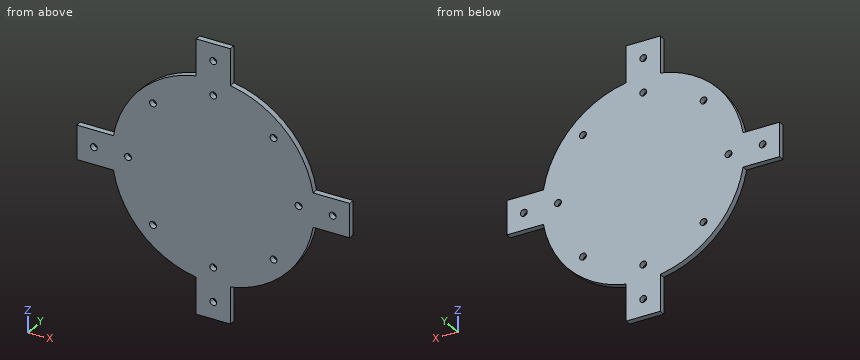
```python
from build123d import *

# Parameters (mm, degrees)
SALIENTE_EXTRUIR1_DEPTH = 3.5
CROQUIS2_R              = 2
CORTAR_EXTRUIR1_DEPTH   = 3.5
MATRIZC1_COUNT          = 8
CORTAR_EXTRUIR2_REACH   = 5.5
CROQUIS4_R              = 2


with BuildPart() as part:
    # Croquis1 → Saliente-Extruir1 (new body)
    with BuildSketch(Plane(origin=(0, 0, 0), x_dir=(1, 0, 0), z_dir=(0, 1, 0))):
        with BuildLine():
            Line((-10, -58.530413525), (-10, -80))
            Line((-10, -80), (10, -80))
            Line((10, -80), (10, -58.530413525))
            ThreePointArc((10, -58.530413525), (41.986958138, -41.986958138), (58.530413525, -10))
            Line((58.530413525, -10), (80, -10))
            Line((80, -10), (80, 10))
            Line((80, 10), (58.530413525, 10))
            ThreePointArc((58.530413525, 10), (41.986958138, 41.986958138), (10, 58.530413525))
            Line((10, 58.530413525), (10, 80))
            Line((10, 80), (-10, 80))
            Line((-10, 80), (-10, 58.530413525))
            ThreePointArc((-10, 58.530413525), (-41.986958138, 41.986958138), (-58.530413525, 10))
            Line((-58.530413525, 10), (-80, 10))
            Line((-80, 10), (-80, -10))
            Line((-80, -10), (-58.530413525, -10))
            ThreePointArc((-58.530413525, -10), (-41.986958138, -41.986958138), (-10, -58.530413525))
        make_face()
    extrude(amount=SALIENTE_EXTRUIR1_DEPTH)

    # Croquis2 → Cortar-Extruir1 (cut)
    with BuildSketch(Plane(origin=(0, 3.5, 0), x_dir=(1, 0, 0), z_dir=(0, 1, 0))):
        with Locations((0, 50)):
            Circle(CROQUIS2_R)
    cortar_extruir1 = extrude(amount=-CORTAR_EXTRUIR1_DEPTH, mode=Mode.SUBTRACT)

    # MatrizC1: Cortar-Extruir1 ×8 about axis
    matrizc1_axis = Axis((0, 0, 0), (0, 1, 0))
    for i in range(1, MATRIZC1_COUNT):
        add(cortar_extruir1.rotate(matrizc1_axis, i * 360 / MATRIZC1_COUNT), mode=Mode.SUBTRACT)

    # Croquis4 → Cortar-Extruir2 (cut, up to next)
    with BuildSketch(Plane(origin=(0, 3.5, 0), x_dir=(1, 0, 0), z_dir=(0, 1, 0)), mode=Mode.PRIVATE) as cortar_extruir2_sk1:
        with Locations((0, 70)):
            Circle(CROQUIS4_R)
    cortar_extruir2_tool1 = extrude(cortar_extruir2_sk1.sketch, amount=-CORTAR_EXTRUIR2_REACH, mode=Mode.PRIVATE) & part.part
    add(cortar_extruir2_tool1.solids().sort_by_distance((0, 3.5, -70))[0], mode=Mode.SUBTRACT)
    # Croquis4 → Cortar-Extruir2 (cut, up to next)
    with BuildSketch(Plane(origin=(0, 3.5, 0), x_dir=(1, 0, 0), z_dir=(0, 1, 0)), mode=Mode.PRIVATE) as cortar_extruir2_sk2:
        with Locations((70, 0)):
            Circle(CROQUIS4_R)
    cortar_extruir2_tool2 = extrude(cortar_extruir2_sk2.sketch, amount=-CORTAR_EXTRUIR2_REACH, mode=Mode.PRIVATE) & part.part
    add(cortar_extruir2_tool2.solids().sort_by_distance((70, 3.5, 0))[0], mode=Mode.SUBTRACT)
    # Croquis4 → Cortar-Extruir2 (cut, up to next)
    with BuildSketch(Plane(origin=(0, 3.5, 0), x_dir=(1, 0, 0), z_dir=(0, 1, 0)), mode=Mode.PRIVATE) as cortar_extruir2_sk3:
        with Locations((0, -70)):
            Circle(CROQUIS4_R)
    cortar_extruir2_tool3 = extrude(cortar_extruir2_sk3.sketch, amount=-CORTAR_EXTRUIR2_REACH, mode=Mode.PRIVATE) & part.part
    add(cortar_extruir2_tool3.solids().sort_by_distance((0, 3.5, 70))[0], mode=Mode.SUBTRACT)
    # Croquis4 → Cortar-Extruir2 (cut, up to next)
    with BuildSketch(Plane(origin=(0, 3.5, 0), x_dir=(1, 0, 0), z_dir=(0, 1, 0)), mode=Mode.PRIVATE) as cortar_extruir2_sk4:
        with Locations((-70, 0)):
            Circle(CROQUIS4_R)
    cortar_extruir2_tool4 = extrude(cortar_extruir2_sk4.sketch, amount=-CORTAR_EXTRUIR2_REACH, mode=Mode.PRIVATE) & part.part
    add(cortar_extruir2_tool4.solids().sort_by_distance((-70, 3.5, 0))[0], mode=Mode.SUBTRACT)


solid = part.part
```
Model file for the job. Use its own axes, mm. Round coordinates to 2 decimals unless told otherwise and drop trailing zeros. Write each loop counter-clockwise with the first axis right and the second up, starting at its lowest first coordinate (ties: lowest second). Pieces come first, ordered by that corner, then holes. Notation, with made-up numbers: M 47.25,-13 L 75.25,-13 A14 cw 75.25,4 Z; hole C -8.75,74.5 d5. An arc over 180 degrees is marked long. Put each result on its own line as item: value.
Item 1: Flat gauge pins, fed straight in: P1, Ø3.5, axis at x = -35.36, z = 35.36, coming from the -Y side; P2, Ø1.8, axis at y = 1, z = -71.5, coming from the -X side; P3, Ø1.8, axis at x = 72.5, y = 2, coming from the +Z side; P4, Ø1, axis at x = -34.5, y = 1, coming from the -Z side. Where does each tip first touch, or does it go through?
Responses:
P1: through
P2: x = -10
P3: z = 10
P4: z = -48.68
Item 2: Cut at B-B (x = 70). List the corners of the cut face in (y, z), and give its area (3 significant figures).
Responses:
outline: M 0,-10 L 3.5,-10 L 3.5,-2 L 0,-2 Z; M 0,2 L 3.5,2 L 3.5,10 L 0,10 Z
area: 56.0 mm²
Item 3: Probe L1, parallel to Z at x = -35, y = 3.2; L2, parallel to X at y = 2.4, z = 0; L3, parallel to X at y = 1.3, z = -70. List the from-to ranges inside material, lowest first. Write a range as from..to.
Responses:
L1: -47.97..-37.32, -33.39..33.39, 37.32..47.97
L2: -80..-72, -68..-52, -48..48, 52..68, 72..80
L3: -10..-2, 2..10
Item 4: Cut at A-A (z = 70). List the corners of the cut face in (x, y), and give its area (3 significant figures).
Responses:
outline: M -10,0 L -2,0 L -2,3.5 L -10,3.5 Z; M 2,0 L 10,0 L 10,3.5 L 2,3.5 Z
area: 56.0 mm²
Item 5: Cut at D-D (x = -14). List the corners of the cut face in (y, z), and give its area (3 significant figures).
Responses:
outline: M 0,-57.7 L 3.5,-57.7 L 3.5,57.7 L 0,57.7 Z
area: 404 mm²
Item 6: Cut at C-C (y = 1.5). State how many separate pieces and enclosed holes the cut face has, and give its area (3 significant figures).
Responses:
separate pieces: 1
enclosed holes: 12
area: 12,600 mm²
